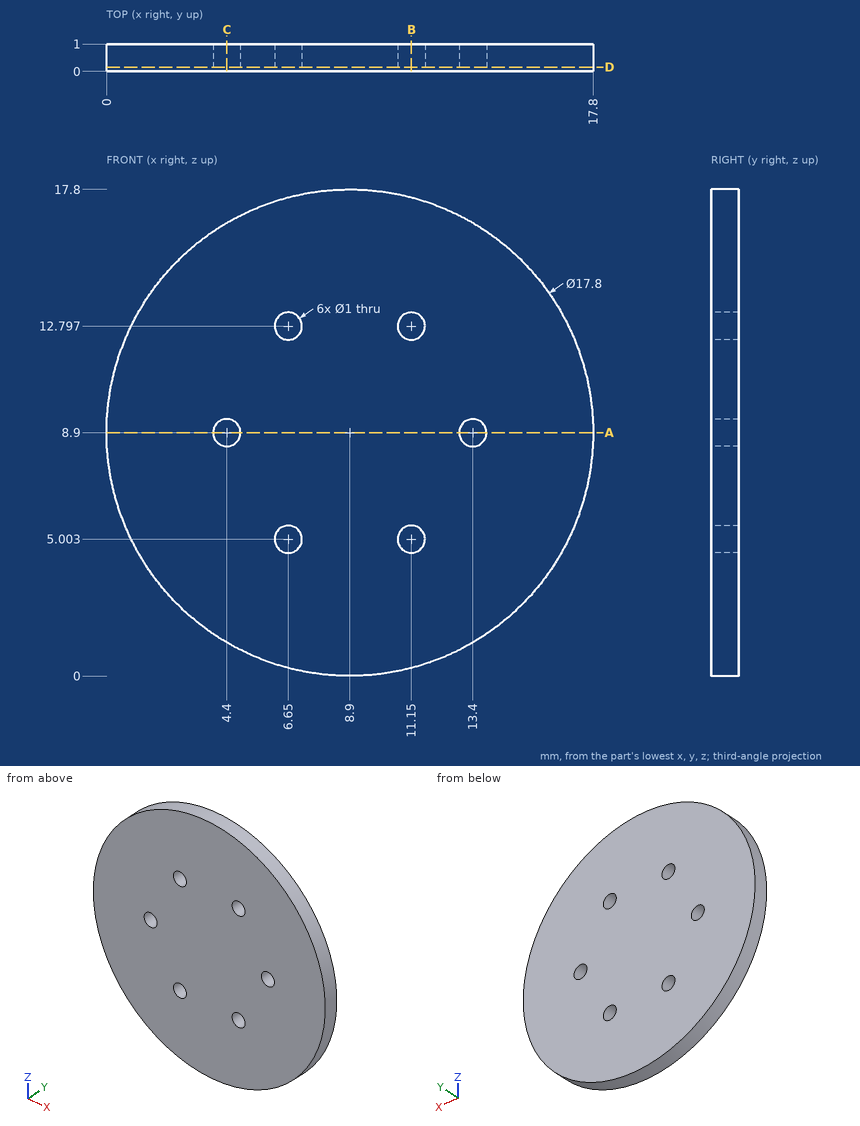
Design review of the part shown in the three views and the two pictorial views. Dimensions are in mm from the part's minimum x, y and z. Round coordinates to 2 decimals unless told otherwise and drop trailing zeros. Loops run counter-clockwise (first coordinate to the right, second up) from the corner with the lowest first, then second, coordinate; pieces in that order, holes last. Notation, with made-up numbers: (43.25, 87.25) - (69.25, 87.25) arc R11 cw to (69.25, 92.25) - close; hole circle Ø11 at (37.25, 11). An arc over 180 degrees is marked (long way). Write each question's results on one line, items separated by ' | '. Start each with the question number.
Q1. Take a section at D-D on y = 0.15. Give the boundary of the cut face in (x, z), plus the area to 3 significant figures.
Q2. Take a section at B-B on x = 11.15. Give the boundary of the cut face in (y, z), plus the area to 3 significant figures.
Q3. Take a section at C-C on x = 4.4. Give the boundary of the cut face in (y, z).
Q4. Take a section at A-A on z = 8.9. Give the boundary of the cut face in (x, y), plus the area to 3 significant figures.
Q5. Wall thickness on line 1 along X through (y, z) = (0.5, 12.5); line 2 along Z through (x, y) = (4, 0.25); line 3 along Z through (x, y) = (4.5, 0.6): over which ranges is each line inside the solid? List them lowest first. Write a range as [from, to].
Data:
1) outline: circle Ø17.8 at (8.9, 8.9); hole circle Ø1 at (4.4, 8.9); hole circle Ø1 at (6.65, 5); hole circle Ø1 at (6.65, 12.8); hole circle Ø1 at (11.15, 5); hole circle Ø1 at (11.15, 12.8); hole circle Ø1 at (13.4, 8.9) | area: 244 mm²
2) outline: (0, 0.29) - (1, 0.29) - (1, 4.5) - (0, 4.5) - close; (0, 5.5) - (1, 5.5) - (1, 12.3) - (0, 12.3) - close; (0, 13.3) - (1, 13.3) - (1, 17.51) - (0, 17.51) - close | area: 15.2 mm²
3) outline: (0, 1.22) - (1, 1.22) - (1, 8.4) - (0, 8.4) - close; (0, 9.4) - (1, 9.4) - (1, 16.58) - (0, 16.58) - close
4) outline: (0, 0) - (3.9, 0) - (3.9, 1) - (0, 1) - close; (4.9, 0) - (12.9, 0) - (12.9, 1) - (4.9, 1) - close; (13.9, 0) - (17.8, 0) - (17.8, 1) - (13.9, 1) - close | area: 15.8 mm²
5) line 1: x = [0.76, 6.25], [7.05, 10.75], [11.55, 17.04] | line 2: z = [1.47, 8.6], [9.2, 16.33] | line 3: z = [1.16, 8.41], [9.39, 16.64]
